from build123d import *

# Parameters (mm, degrees)
F0_R      = 6.35
F1_DEPTH  = 15.24
F2_R      = 8.89
F3_DEPTH  = 2.54
F4_R      = 1.26999
F5_R      = 8.89
F6_DEPTH  = 2.54
F7_R      = 1.26999
F8_R      = 6.35
F9_DEPTH  = 19.05
F10_R     = 6.35
F11_DEPTH = 14.097
F12_SIZE  = 1.27


# Not quite as in the source:
# - a fillet or chamfer is up to 0.001 mm smaller than in the source, because OpenCascade refuses the exact size


with BuildPart() as f1:
    # F0 (on Right) → F1 (new body)
    with BuildSketch(Plane.YZ):
        with Locations((0, 182.4067449291)):
            Circle(F0_R)
    extrude(amount=F1_DEPTH)

    # F2 (on face) → F3 (join)
    with BuildSketch(Plane(origin=(0, 0, 0), x_dir=(0, -1, 0), z_dir=(-1, 0, 0))):
        with Locations((0, 182.4067449291)):
            Circle(F2_R)
    extrude(amount=F3_DEPTH)

    # F4 (radius 1.27 in the source; OpenCascade refuses exactly that, so slightly less here)
    f4_edges = [f1.edges().sort_by_distance(p)[0] for p in [
        (-1.27, -8.89, 182.406745),
        (0, 8.89, 182.406745),
        (-2.54, 8.89, 182.406745),
    ]]
    fillet(f4_edges, radius=F4_R)

    # F5 (on face) → F6 (join)
    with BuildSketch(Plane.YZ.offset(15.24)):
        with Locations((0, 182.4067449291)):
            Circle(F5_R)
    extrude(amount=F6_DEPTH)

    # F7 (radius 1.27 in the source; OpenCascade refuses exactly that, so slightly less here)
    f7_edges = [f1.edges().sort_by_distance(p)[0] for p in [
        (16.51, 8.89, 182.406745),
        (15.24, -8.89, 182.406745),
        (17.78, -8.89, 182.406745),
    ]]
    fillet(f7_edges, radius=F7_R)



with BuildPart() as f9:
    # F8 (on Front) → F9 (new body, symmetric)
    with BuildSketch(Plane.XZ):
        with Locations((34.29, 182.4067449291)):
            Circle(F8_R)
    extrude(amount=F9_DEPTH, both=True)


with BuildPart() as f1_1:
    add(f1.part)

    add(f9.part)  # F11 merges F9
    # F10 (on face) → F11 (join)
    with BuildSketch(Plane.YZ.offset(17.78)):
        with Locations((0, 182.4067449291)):
            Circle(F10_R)
    extrude(amount=F11_DEPTH)

    # F12
    f12_edges = [f1_1.edges().sort_by_distance(p)[0] for p in [
        (27.94, -19.05, 182.406745),
        (27.94, 19.05, 182.406745),
    ]]
    chamfer(f12_edges, length=F12_SIZE)


with BuildPart() as f1_2:
    # F14: moved
    add(f1_1.part.moved(Location((-15.24, 0, -182.4067449291))))


solid = f1_2.part
Read the model definition and answer for the solid it produces. Units are mm, in the model's axes. A direction names the side the tool comes from. Round coordinates to 2 decimals unless told otherwise and drop trailing zeros. Order: outer loops, then holes, each group sorted by start corner. A loop starts at its lowest first (then second) coordinate and runs counter-clockwise, first axis right, second up.
1) Straight lines are drawn through the part: L1, parallel to X at y = -2.5, z = 8; L2, parallel to X at y = -6.5, z = -2.5; L3, parallel to X at y = -4, z = 6.75. For each, find the intervals that lie inside material, in ascending order.
2) Flat-ended cylindrical pins translate along their axes: pin 1 (4 mm diameter, centred on y = -14.5, z = -2.5, fed in from -X); pin 2 (7.5 mm diameter, centred on y = 2, z = -2.5, fed in from +X); pin 3 (12 mm diameter, centred on x = 10, y = -11.5, fed in from +Z); pin 4 (2 mm diameter, centred on y = -9, z = 2, fed in from -X). Find the tip coordinate at first contact, or state that the pin passes through.
3) The mould has two halves that part along X. Classify faces 1 (the face through (19, 19.05, 0)), 2 (the face through (-17.78, 0, 0)), 3 (the face through (2.54, -3, 6)): released by +X, released by -X, zero draft, split by the parting line, or undercut.
4) The part is cut by section C-C on x = 19.05. Write down the section's boundary in (y, z), plus the area to 3 significant figures.
5) The part is cut by section D-D on y = 7. Give the number of separate pieces and of enclosed holes in the cut face, plus the area to 3 significant figures.
6) For faces 4 (the face through (24.916, -0.249, -2.432)), 5 (the face through (19, -19.05, 0)), determine the directions among +Z, -Z, +X, -X, +Y, -Y from which every point of the face is accessible in a straight line to the end or side of a thin tool.
Resolved:
1. L1: x = -17.53 to -15.49, 0.25 to 2.29
1. L2: x = -17.78 to -15.24, 0 to 2.54, 13.21 to 24.89
1. L3: x = -17.76 to -15.26, 0.02 to 2.52
2. pin 1: stops at x = 12.72
2. pin 2: stops at x = 25.4
2. pin 3: stops at z = 5.57
2. pin 4: stops at x = -17.63
3. face 1: zero draft
3. face 2: released by -X
3. face 3: undercut
4. outline: (-19.05, -5.08) - (-17.78, -6.35) - (17.78, -6.35) - (19.05, -5.08) - (19.05, 5.08) - (17.78, 6.35) - (-17.78, 6.35) - (-19.05, 5.08) - close
4. area: 481 mm2
5. separate pieces: 3
5. enclosed holes: 0
5. area: 178 mm2
6. face 4: none
6. face 5: +Z, -Z, +X, -X, -Y
